from build123d import *

# Parameters (mm, degrees)
SKETCH1_W               = 45
SKETCH1_H               = 12
BOSS_EXTRUDE1_DEPTH     = 2
FILLET1_R               = 3
FILLET15_R              = 0.5
CUT_EXTRUDE2_DEPTH      = 46.442271187
CUT_EXTRUDE2_DEPTH_BACK = 15
SKETCH11_W              = 4.5
SKETCH11_H              = 4
BOSS_EXTRUDE3_DEPTH     = 3
SKETCH14_R              = 1.5
CUT_EXTRUDE4_DEPTH      = 26.985573053
FILLET17_R              = 1


with BuildPart() as part:
    # Sketch1 → Boss-Extrude1 (new, symmetric)
    with BuildSketch(Plane(origin=(0, 0, 0), x_dir=(1, 0, 0), z_dir=(0, 1, 0))):
        Rectangle(SKETCH1_W, SKETCH1_H)
    extrude(amount=BOSS_EXTRUDE1_DEPTH, both=True)

    # Sketch2 → Cut-Revolve2 (revolve, cut)
    with BuildSketch(Plane.XY):
        with BuildLine():
            Line((-17, 2), (-17, -2))
            Line((-17, -2), (-20.5, -2))
            ThreePointArc((-20.5, -2), (-21.031128874, 0), (-20.5, 2))
            Line((-20.5, 2), (-17, 2))
        make_face()
    revolve(axis=Axis((-17, 2, 0), (0, -1, 0)), mode=Mode.SUBTRACT)

    # Fillet1
    fillet1_edges = [part.edges().sort_by_distance(p)[0] for p in [
        (-22.5, 0, 6),
        (-22.5, 0, -6),
    ]]
    fillet(fillet1_edges, radius=FILLET1_R)

    # Fillet15
    fillet15_edges = [part.edges().sort_by_distance(p)[0] for p in [
        (-13.5, 2, 0),
        (-13.5, -2, 0),
    ]]
    fillet(fillet15_edges, radius=FILLET15_R)

    # Sketch11 → Cut-Extrude2 (cut, two sides: drawn at the far end of the back side and taken through both)
    with BuildSketch(Plane(origin=(22.5, 0, 0), x_dir=(0, 0, -1), z_dir=(1, 0, 0)).offset(-CUT_EXTRUDE2_DEPTH_BACK)):
        Rectangle(SKETCH11_W, SKETCH11_H)
    extrude(amount=CUT_EXTRUDE2_DEPTH + CUT_EXTRUDE2_DEPTH_BACK, mode=Mode.SUBTRACT)

    # Sketch13 → Boss-Extrude3 (add)
    with BuildSketch(Plane(origin=(0, 2, 0), x_dir=(1, 0, 0), z_dir=(0, 1, 0))):
        Polygon((22.5, 2.25), (7.5, 2.25), (7.5, -2.25), (22.5, -2.25), (22.5, -6), (1.5, -6), (1.5, -2.5), (1.5, 2.5), (1.5, 6), (22.5, 6), align=None)
    extrude(amount=BOSS_EXTRUDE3_DEPTH)

    # Sketch14 → Cut-Extrude4 (cut, through all)
    with BuildSketch(Plane(origin=(0, 0, -6), x_dir=(-1, 0, 0), z_dir=(0, 0, -1))):
        with Locations((-17.5, 1.5)):
            Circle(SKETCH14_R)
        with Locations((-10.5, 1.5)):
            Circle(SKETCH14_R)
    extrude(amount=-CUT_EXTRUDE4_DEPTH, mode=Mode.SUBTRACT)

    # Fillet17
    fillet17_edges = [part.edges().sort_by_distance(p)[0] for p in [
        (1.5, 2, 0),
        (1.5, 5, 0),
    ]]
    fillet(fillet17_edges, radius=FILLET17_R)


solid = part.part
Read the model definition and answer for the solid it produces. Units are mm, in the model's axes. A direction names the side the tool comes from. Coordinates: 2 decimals unless noted, no trailing zeros. Loops run counter-clockwise (first coordinate to the right, second up) from the corner with the lowest first, then second, coordinate; pieces in that order, holes last. Notation, with made-up numbers: (7, 28) -> (40, 28) arc R22 ccw to (40, 61) -> close; hole circle Ø5 at (76.5, -33.75). An arc over 180 degrees is marked (long way). Write item = value, one per line. Start each with the question number.
1) Given P1, Ø1.5, axis at x = -8.5, z = 0.5, coming from the +Y side; P2, Ø0.5, axis at y = 3.5, z = 1, coming from the -X side; P3, Ø3.5, axis at y = 0, z = 0, coming from the +X side, each flat-ended and moving along its own axis, determine where each tip first touches the part or whether it passes through.
2) For faces 1 (the face through (-9, 2, 0)), 2 (the face through (22.5, 1, 4)), 3 (the face through (15, 1, -2.25)), determine the directions among +Z, -Z, +X, -X, +Y, -Y from which every point of the face is accessible in a straight line to the end or side of a thin tool.
3) The part is cut by section B-B, the plane z = 3.5. State how many separate pieces and enclosed holes the cut face has, plus the area to 3 significant figures.
4) Find the intervals of material crossed by L1, parallel to Y at x = 17.5, z = 4.6; L2, parallel to Z at x = 9, y = 2.5; L3, parallel to Z at x = -14.5, y = 1, in increasing order. Write a range as from..to.
5) The part is cut by section C-C, the plane x = -3. Determine the outline of the cut face in (y, z), plus the area to 3 significant figures.
6) The part is cut by section A-A, the plane x = 10.5. Determine the outline of the cut face in (y, z).
7) The mould has two halves that part along Y. Classify faces 4 (the face through (15, 1, 2.25)), 5 (the face through (12, 1.57, -4.15)), 6 (the face through (0, -2, 0)): pulls with the +Y half, pulls with the -Y half, needs draft (parallel to the pull), parting line crosses it, or undercut.
Result:
q1.P1 = 2
q1.P2 = 1.5
q1.P3 = 7.5
q2.face_1 = +Z, -Z, -X, +Y
q2.face_2 = +Z, -Z, +X, +Y, -Y
q2.face_3 = +X, +Y, -Y
q3.separate_pieces = 2
q3.enclosed_holes = 2
q3.area = 215 mm²
q4.L1 = -2..0, 3..5
q4.L2 = -6..-2.25, 2.25..6
q4.L3 = -6..-3, 3..6
q5.outline = (-2, -6) -> (2, -6) -> (2, 6) -> (-2, 6) -> close
q5.area = 48.0 mm²
q6.outline = (-2, -6) -> (0, -6) -> (0, -2.25) -> (-2, -2.25) -> close; (-2, 2.25) -> (0, 2.25) -> (0, 6) -> (-2, 6) -> close; (3, -6) -> (5, -6) -> (5, -2.25) -> (3, -2.25) -> close; (3, 2.25) -> (5, 2.25) -> (5, 6) -> (3, 6) -> close
q7.face_4 = needs draft
q7.face_5 = undercut
q7.face_6 = pulls with the -Y half
